The model under review builds one solid part; all positions refer to its coordinate system, in mm. A direction names the side the tool comes from. Round coordinates to 2 decimals unless told otherwise and drop trailing zeros. Write each loop counter-clockwise with the first axis right and the second up, starting at its lowest first coordinate (ties: lowest second). Pieces come first, ordered by that corner, then holes. Notation, with made-up numbers: M 45.25,-3.5 L 96.25,-3.5 A37 cw 96.25,33.5 Z; hole C 35.5,37.25 d10. An arc over 180 degrees is marked long. One line per item, written item: value. Start each with the question number.
1) Tool access review of faces 5 (the face through (-0.03, -5.85, -0.79)), 6 (the face through (-3, 0, 1)): name each direction out of +Z, -Z, +X, -X, +Y, -Y from which nothing blocks a thin tool from reaching the whole face with its end or side.
2) Take a section at B-B, the plane y = -2.5. Write out the cut boundary in (x, z) (3 decimals).
3) Take a section at D-D, the plane y = 3. Write out the cut boundary in (x, z) (3 decimals).
4) Take a section at C-C, the plane x = 0. Write out the cut boundary in (y, z) (3 decimals).
5) For P1, Ø1, axis at y = 4.5, z = 0, coming from the +X side; P2, Ø1.1, axis at x = 0, z = 0, coming from the +Y side, all flat-tipped, find the tip position at first contact; note any pin that passes through.
6) Wall thickness on probe 1 along X at (y, z) = (3, 0) (3 decimals); probe 2 along Z at (x, y) = (-0.25, -2.5); probe 3 along X at (y, z) = (-5.4, 0) (3 decimals): over which ranges is each line inside the solid? List them lowest first.
7) Take a section at A-A, the plane z = 0. Write out the cut boundary in (x, y) (3 decimals).
8) Mouldability with a two-part tool opening along Z and no side actions: class faces 1 (the face through (0, -2, 3.5)), 2 (the face through (4.475, -1.595, -0.056)), 3 (the face through (1, 5.95, -1)), 4 (the face through (0.903, 0.752, -0.201)) as +Z half, -Z half, draft (parallel to the pull), parting line (faces both ways), or undercut.
from build123d import *

# Parameters (mm, degrees)
CUT_EXTRUDE1_REACH = 10.721
SKETCH2_W          = 5.576961538
SKETCH2_H          = 0.975
CHAMFER1_SIZE      = 0.5
CHAMFER2_SIZE      = 0.15


with BuildPart() as part:
    # Sketch1 → Revolve1 (revolve)
    with BuildSketch(Plane(origin=(0, 0, 0), x_dir=(0, 0, -1), z_dir=(1, 0, 0)), mode=Mode.PRIVATE) as revolve1_sk:
        Polygon((0.925, -4.438709677), (0.925, 5.95), (3, 5.95), (3, 0), (4.475, 0), (4.475, -3), (0.6, -6), (0.2, -6), (0.2, -5), align=None)
    revolve(revolve1_sk.sketch.rotate(Axis((0, 16.051202931, 0), (0, -1, 0)), 180), axis=Axis((0, 16.051202931, 0), (0, -1, 0)))

    # Cut-Extrude1: up to this cone (the profile starts inside it)
    cut_extrude1_end = Plane(origin=(0, 0, 0), z_dir=(0, 1, 0)).offset(-6.464515129) * Cone(1.292e-06, 33.629208333, 26.035515129, align=(Align.CENTER, Align.CENTER, Align.MIN), mode=Mode.PRIVATE)
    # Sketch2 → Cut-Extrude1 (cut, up to the surface)
    with BuildSketch(Plane(origin=(0, 0, 0), x_dir=(1, 0, 0), z_dir=(0, 1, 0)), mode=Mode.PRIVATE) as cut_extrude1_sk1:
        with Locations((0, -3.9875)):
            Rectangle(SKETCH2_W, SKETCH2_H)
    cut_extrude1_tool1 = extrude(cut_extrude1_sk1.sketch, amount=-CUT_EXTRUDE1_REACH, mode=Mode.PRIVATE) & cut_extrude1_end
    add(cut_extrude1_tool1.solids().sort_by_distance((0, 0, 3.9875))[0], mode=Mode.SUBTRACT)
    # Sketch2 → Cut-Extrude1 (cut, up to the surface)
    with BuildSketch(Plane(origin=(0, 0, 0), x_dir=(1, 0, 0), z_dir=(0, 1, 0)), mode=Mode.PRIVATE) as cut_extrude1_sk2:
        with Locations((0, 3.9875)):
            Rectangle(SKETCH2_W, SKETCH2_H)
    cut_extrude1_tool2 = extrude(cut_extrude1_sk2.sketch, amount=-CUT_EXTRUDE1_REACH, mode=Mode.PRIVATE) & cut_extrude1_end
    add(cut_extrude1_tool2.solids().sort_by_distance((0, 0, -3.9875))[0], mode=Mode.SUBTRACT)

    # Chamfer1
    chamfer1_edges = [part.edges().sort_by_distance(p)[0] for p in [
        (0, 5.95, -3),
    ]]
    chamfer(chamfer1_edges, length=CHAMFER1_SIZE)

    # Chamfer2
    chamfer2_edges = [part.edges().sort_by_distance(p)[0] for p in [
        (-4.475, 0, 0),
        (4.475, 0, 0),
        (0, 5.95, -0.925),
    ]]
    chamfer(chamfer2_edges, length=CHAMFER2_SIZE)


solid = part.part
Checked values:
1. face 5: -Y
1. face 6: +Y
2. outline: M -2.788,-3.5 L 2.788,-3.5 A4.475 ccw 2.788,3.5 L -2.788,3.5 A4.475 ccw Z; hole C 0,0 d1.85
3. outline: C 0,0 d6; hole C 0,0 d1.85
4. outline: M -6,-0.6 L -3.755,-3.5 L 0,-3.5 L 0,-3 L 5.45,-3 L 5.95,-2.5 L 5.95,-1.075 L 5.8,-0.925 L -4.439,-0.925 L -5,-0.2 L -6,-0.2 Z; M -6,0.2 L -5,0.2 L -4.439,0.925 L 5.8,0.925 L 5.95,1.075 L 5.95,2.5 L 5.45,3 L 0,3 L 0,3.5 L -3.755,3.5 L -6,0.6 Z
5. P1: stops at x = 3
5. P2: stops at y = -4.73
6. probe 1: x = -3 to -0.925, 0.925 to 3
6. probe 2: z = -3.5 to -0.89, 0.89 to 3.5
6. probe 3: x = -1.375 to -0.2, 0.2 to 1.375
7. outline: M -4.475,-3 L -0.6,-6 L -0.2,-6 L -0.2,-5 L -0.925,-4.439 L -0.925,5.8 L -1.075,5.95 L -2.5,5.95 L -3,5.45 L -3,0 L -4.325,0 L -4.475,-0.15 Z; M 0.2,-6 L 0.6,-6 L 4.475,-3 L 4.475,-0.15 L 4.325,0 L 3,0 L 3,5.45 L 2.5,5.95 L 1.075,5.95 L 0.925,5.8 L 0.925,-4.439 L 0.2,-5 Z
8. face 1: +Z half
8. face 2: parting line
8. face 3: draft
8. face 4: undercut
